Source: CAD feature listing. Evaluate the final solid. Frame: model axes, mm. Face numbers are marked on the shaded views. A direction names the side the tool comes from. Coordinates: 2 decimals unless noted, no trailing zeros. Loops run counter-clockwise (first coordinate to the right, second up) from the corner with the lowest first, then second, coordinate; pieces in that order, holes last. Notation, with made-up numbers: (46, -4.75) - (98, -4.75) arc R29 cw to (98, 29.25) - close; hole circle Ø10 at (53, 72.5). An arc over 180 degrees is marked (long way). Use one line per item in the form item = value. Start each with the question number.
from build123d import *

# Parameters (mm, degrees)
F0_W      = 82.2246223688
F0_H      = 71.0700303316
F1_DEPTH  = 1000
F2_DEPTH  = 675
F3_DEPTH  = 675
F4_W      = 383.3865523338
F4_H      = 348.4983026981
F5_DEPTH  = 25
F6_DEPTH  = 84.39
F7_DEPTH  = 49.5
F9_DEPTH  = 25
F10_DEPTH = 975
F11_T     = -18


with BuildPart() as f1:
    # F0 (on Top) → F1 (new body)
    with BuildSketch(Plane.XY):
        with Locations((41.1123111844, -35.5350151658)):
            Rectangle(F0_W, F0_H)
    extrude(amount=F1_DEPTH)

    # F2 (add): a face of the model
    f2_faces = [f1.faces().sort_by_distance(p)[0] for p in [
        (0, -35.5350151658, 500),
    ]]
    extrude(f2_faces, amount=-F2_DEPTH)

    # F3 (add): a face of the model
    f3_faces = [f1.faces().sort_by_distance(p)[0] for p in [
        (337.5, 0, 500),
    ]]
    extrude(f3_faces, amount=-F3_DEPTH)

    # F4 (on face) → F5 (cut)
    with BuildSketch(Plane.XY.offset(1000)):
        with Locations((191.6932761669, -500.7508486509)):
            Rectangle(F4_W, F4_H)
    extrude(amount=-F5_DEPTH, mode=Mode.SUBTRACT)

    # F6 (add): a face of the model
    f6_faces = [f1.faces().sort_by_distance(p)[0] for p in [
        (383.3865523338, -500.7508486509, 987.5),
    ]]
    extrude(f6_faces, amount=F6_DEPTH)

    # F7 (add): a face of the model
    f7_faces = [f1.faces().sort_by_distance(p)[0] for p in [
        (149.4982761669, -326.5016973019, 987.5),
    ]]
    extrude(f7_faces, amount=F7_DEPTH)

    # F8 (on face) → F9 (join)
    with BuildSketch(Plane.XY.offset(975)):
        Polygon((0, -376.0016973019), (298.9965523338, -675), (298.9965523338, -376.0016973019), align=None)
    extrude(amount=F9_DEPTH)

    # F10 (cut): a face of the model
    f10_faces = [f1.faces().sort_by_distance(p)[0] for p in [
        (99.6655174446, -575.3338991006, 975),
    ]]
    extrude(f10_faces, amount=-F10_DEPTH, mode=Mode.SUBTRACT)

    # F11
    f11_openings = [f1.faces().sort_by_distance(p)[0] for p in [
        (149.498276, -525.500849, 500),
    ]]
    offset(amount=F11_T, openings=f11_openings)


solid = f1.part
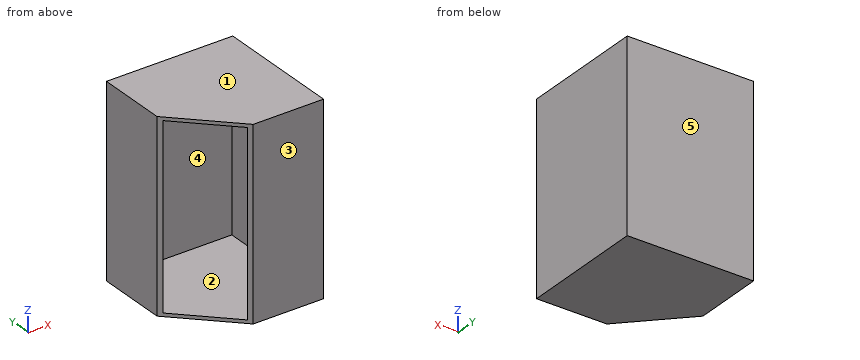
(1) Cut plane D-D, the plane y = -600.5. Output: boundary loops of the cut face in (x, z).
(2) Mould query, pull axis Y, two halves, no side actions, for the marked faces 1, 2 and 3. Classes: +Y half, -Y half, draft (parallel to the pull), parting line (faces both ways), or undercut.
(3) Cut plane B-B, the plane y = -205. Output: boundary loops of the cut face in (x, z), plus the area to 3 significant figures.
(4) Cut plane C-C, the plane z = 70. Output: boundary loops of the cut face in (x, y), plus the area to 3 significant figures.
(5) Contact query for a flat-ended pin moving along its axis: pin 1 (10 mm diameter, centred on y = -528.5, z = 565.5, fed in from -X). Output: stop coordinate, or through.
(6) Access query for the marked faces 4 and 5. Directions: +Z, -Z, +X, -X, +Y, -Y. A direction counts if a zero-diameter tool reaches every point of the face in a straight line with its end or side. Return the directions, or none.
(7) Material intervals for line 1 (Z direction, x = 79, y = -214.5); line 2 (Y direction, x = 434, z = 444.5); line 3 (X direction, y = -28, z = 825), sorted ascending.
(8) Cut plane A-A, the plane x = 516. Output: boundary loops of the cut face in (y, z).
Recorded:
q1.outline = (224.5, 0) - (675, 0) - (675, 1000) - (224.5, 1000) - (224.5, 982) - (657, 982) - (657, 18) - (224.5, 18) - close
q2.face_1 = draft
q2.face_2 = undercut
q2.face_3 = -Y half
q3.outline = (0, 0) - (675, 0) - (675, 1000) - (0, 1000) - close; hole (18, 18) - (657, 18) - (657, 982) - (18, 982) - close
q3.area = 59,000 mm²
q4.outline = (0, -376) - (18, -394) - (18, -18) - (657, -18) - (657, -657) - (281, -657) - (299, -675) - (675, -675) - (675, 0) - (0, 0) - close
q4.area = 37,200 mm²
q5.pin_1 = 657
q6.face_4 = none
q6.face_5 = +Z, -Z, +X, -X, +Y
q7.line_1 = 0 to 18, 982 to 1000
q7.line_2 = -675 to -657, -18 to 0
q7.line_3 = 0 to 18, 657 to 675
q8.outline = (-675, 0) - (0, 0) - (0, 1000) - (-675, 1000) - close; hole (-657, 18) - (-18, 18) - (-18, 982) - (-657, 982) - close
